Geometry: see drawing. Coordinates: mm, zero at the bounding-box minimum. A direction names the side the tool comes from. Coordinates: 2 decimals unless noted, no trailing zeros. Order: outer loops, then holes, each group sorted by start corner. A loop starts at its lowest first (then second) coordinate and runs counter-clockwise, first axis right, second up. Notation, with made-up numbers: (-37, 14.5) -> (-5, 14.5) arc R35 ccw to (-5, 52.5) -> close; hole circle Ø1 at (59.5, 17.25). An arc over 180 degrees is marked (long way). Use CSV: the item, a comma, the result in double quotes. Start each with the question number.
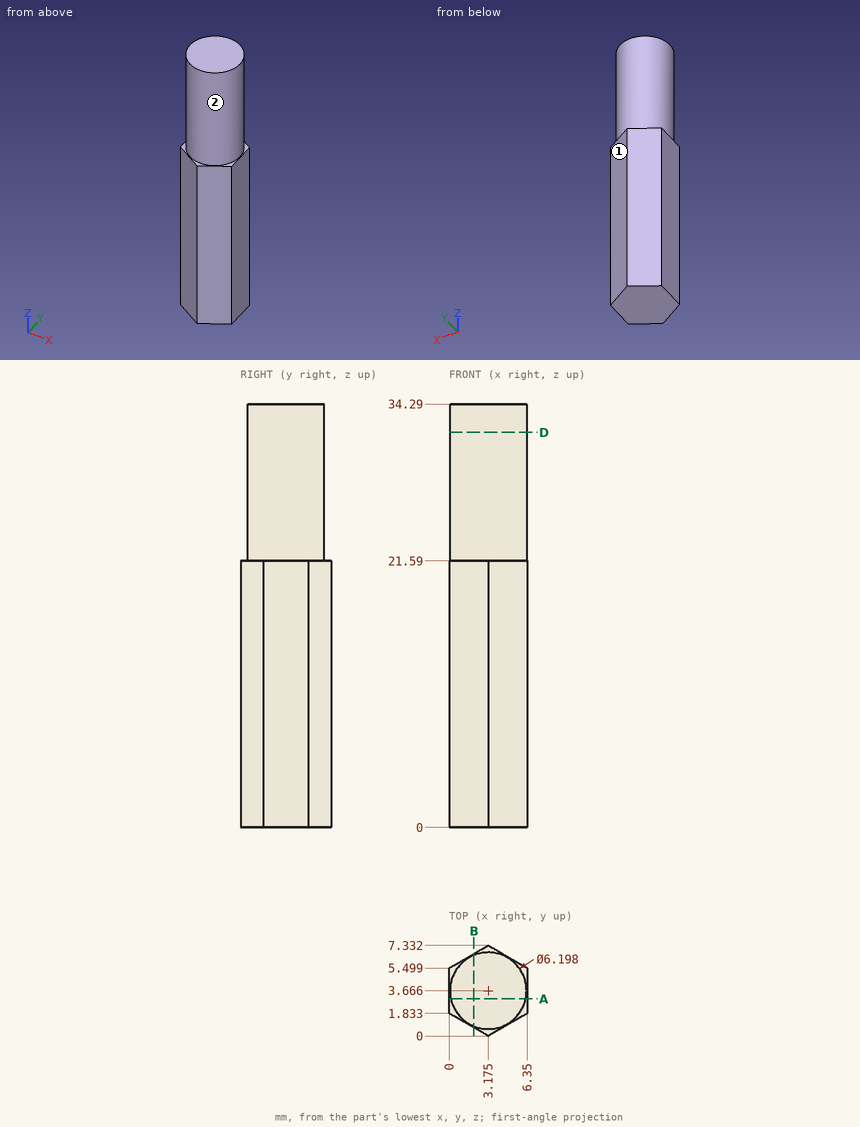
(1) Section B-B (x = 2). Return loops of the section in (y, z).
(2) First-contact query: pin 1 (2 mm diameter, centred on x = 5, y = 6.5, fed in from +Z). Flat tip, straight axial feed; report the tip coordinate or a pass-through.
(3) Access query for the marked faces 1 and 2. Directions: +Z, -Z, +X, -X, +Y, -Y. A direction counts if a zero-diameter tool reaches every point of the face in a straight line with its end or side. Return the directions, or none.
(4) Line query: line 1 (X direction, y = 1, z = 11.5) (1 decimal); line 2 (X direction, y = 4.25, z = 32.5); line 3 (Y direction, x = 1, z = 21) (1 decimal). Output: solid intervals per line, ascending. Write a range as from..to.
(5) Section A-A (y = 3). Return loops of the section in (x, z).
(6) Section D-D (z = 32). Return loops of the section in (x, y) (1 decimal), then the cut area to 3 significant figures.
Check sheet entries:
1,outline,"(0.68, 0) -> (6.65, 0) -> (6.65, 21.59) -> (6.53, 21.59) -> (6.53, 34.29) -> (0.8, 34.29) -> (0.8, 21.59) -> (0.68, 21.59) -> close"
2,pin 1,"stops at z = 34.29"
3,face 1,"+Z, -Z, +X, +Y"
3,face 2,"+Z"
4,line 1,"x = 1.4..4.9"
4,line 2,"x = 0.13..6.22"
4,line 3,"y = 1.3..6.1"
5,outline,"(0, 0) -> (6.35, 0) -> (6.35, 21.59) -> (6.2, 21.59) -> (6.2, 34.29) -> (0.15, 34.29) -> (0.15, 21.59) -> (0, 21.59) -> close"
6,outline,"circle Ø6.2 at (3.2, 3.7)"
6,area,"30.2 mm^2"
